Read the model definition and answer for the solid it produces. Units are mm, in the model's axes. A direction names the side the tool comes from. Give positions to 0.01 mm unless a question says otherwise; leave off trailing zeros. Order: outer loops, then holes, each group sorted by start corner. A loop starts at its lowest first (then second) coordinate and runs counter-clockwise, first axis right, second up. Notation, with made-up numbers: (77, 55) - (134, 55) arc R18 ccw to (134, 74) - close; hole circle Ø11 at (81.25, 71.25). An arc over 180 degrees is marked (long way). Use a Markdown table: item, result. Add a question column.
1. A cutting plane is placed at C-C on z = 39. Determine the outline of the cut face in (x, y), and give its area (3 significant figures).
2. Flat-ended cylindrical pins translate along their axes: P1, Ø2.5, axis at y = 5.5, z = 53.5, coming from the -X side; P2, Ø3, axis at x = 59, z = 24, coming from the +Y side; P3, Ø2, axis at x = 76.5, z = 18.5, coming from the +Y side. Find the tip coordinate at first contact, or state that the pin passes through.
3. A cutting plane is placed at D-D on y = 1.5. State how many separate pieces and enclosed holes the cut face has, and give its area (3 significant figures).
4. For a pull along X with two mould halves and no side action, classify faces 1 (the cylindrical face through (75.3, 5.3, 16.9)), 2 (the flat face through (2.487, 3, 2)), 3 (the flat face through (87.17, 3, 50)) as released by +X, released by -X, zero draft, split by the parting line, or undercut.
5. A cutting plane is placed at A-A on z = 25. Determine the outline of the cut face in (x, y).
6. A cutting plane is placed at B-B on x = 69. Determine the outline of the cut face in (y, z), and give its area (3 significant figures).
7. Consider L1, parallel to X at y = 1.5, z = 26; L2, parallel to Z at x = 14.5, y = 3; L3, parallel to X at y = 4.25, z = 18. Determine where each line is inside the solid, lowest interval first.
8. Which of the six approach directions +Z, -Z, +X, -X, +Y, -Y give full straight-line access (tool end or side, diameter ignored) to faces 4 (the flat face through (-27, 3, 46.102)), 5 (the flat face through (138.027, 3, 26)), 6 (the flat face through (87.17, 3, 2)), 7 (the flat face through (84.13, 3.13, 56.51)), 8 (the cylindrical face through (22.38, 3.92, 51.01))?
Autodesk Inventor part; units mm, degrees
ref_plane "YZ Plane" through (0, 0, 0) normal (1, 0, 0) x (0, 1, 0)
ref_plane "XZ Plane" through (0, 0, 0) normal (0, 1, 0) x (-1, 0, 0)
ref_plane "XY Plane" through (0, 0, 0) normal (0, 0, 1) x (1, 0, 0)
sketch "Sketch1" plane through (0, 0, 0) normal (0, 1, 0) x (-1, 0, 0)
  line L0 (-41.4486, 0) -> (-10.4831, 0)
  line L1 (-10.4831, 0) -> (-10.4831, 53.4636)
  line L2 (-10.4831, 53.4636) -> (-41.4486, 53.4636)
  line L3 (-41.4486, 53.4636) -> (-41.4486, 0)
  line L4 (-79.1688, 53.4636) -> (-87.1698, 53.4636)
  line L5 (-87.1698, 53.4636) -> (-87.1698, 0)
  line L6 (-87.1698, 0) -> (-79.1688, 0)
  line L7 (-79.1688, 0) -> (-79.1688, 53.4636)
  line L8 (-87.1698, 53.4636) -> (-2.487, 53.4636)
  line L9 (-2.487, 53.4636) -> (-2.487, 59.4685)
  line L10 (-2.487, 59.4685) -> (-87.1698, 59.4685)
  line L11 (-87.1698, 59.4685) -> (-87.1698, 53.4636)
  line L12 (-87.1698, 0) -> (-2.487, 0)
  line L13 (-2.487, 0) -> (-2.487, -7.9038)
  line L14 (-2.487, -7.9038) -> (-87.1698, -7.9038)
  line L15 (-87.1698, -7.9038) -> (-87.1698, 0)
  line L16 (-87.1698, -7.9038) -> (-2.487, -7.9038)
  line L17 (-2.487, -7.9038) -> (-2.487, 59.4685)
  line L18 (-2.487, 59.4685) -> (-87.1698, 59.4685)
  line L19 (-87.1698, 59.4685) -> (-87.1698, -7.9038)
  line L20 (-2.487, -7.9038) -> (-2.487, 25.802)
  line L21 (-2.487, 25.802) -> (-2.487, 59.4685)
  point P0 (0, 0)
  dimension "d0" = 8.001
  dimension "d1" = 33.7058
extrude "Extrusion1" add sketch "Sketch1" along normal blind 6.35
sketch "Sketch3" plane through (0, 6.35, 0) normal (0, 1, 0) x (1, 0, 0)
  line L0 (10.5148, -0.1125) -> (75.0308, -0.1125)
  line L1 (75.0308, -0.1125) -> (76.5548, -1.6365)
  line L2 (76.5548, -1.6365) -> (76.5548, -13.003)
  line L3 (76.5997, -13.1114) -> (79.0948, -15.6065)
  line L4 (79.0948, -15.6065) -> (79.0948, -48.3725)
  line L5 (79.0948, -48.3725) -> (76.5997, -50.8676)
  line L6 (76.5548, -50.976) -> (76.5548, -53.4525)
  line L7 (76.5548, -53.4525) -> (10.5148, -53.4525)
  line L8 (10.5148, -53.4525) -> (10.5148, -0.1125)
  line L9 (77.3168, -12.7509) -> (77.3168, -1.3209)
  line L10 (77.3168, -1.3209) -> (75.3465, 0.6495)
  line L11 (75.3465, 0.6495) -> (9.7528, 0.6495)
  line L12 (9.7528, 0.6495) -> (9.7528, -54.2145)
  line L13 (9.7528, -54.2145) -> (77.3168, -54.2145)
  line L14 (77.3168, -54.2145) -> (77.3168, -51.2282)
  line L15 (77.3168, -51.2282) -> (79.8568, -48.6882)
  line L16 (79.8568, -48.6882) -> (79.8568, -15.2909)
  line L17 (79.8568, -15.2909) -> (77.3168, -12.7509)
  point P0 (0, 0)
  dimension "d4" = 0.762
  dimension "d5" = 0.762
  dimension "d6" = 0.762
  dimension "d7" = 0.762
  dimension "d8" = 0.762
  dimension "d9" = 0.762
extrude "Extrusion2" cut sketch "Sketch3" against normal blind 3
sketch "Sketch4" plane through (0, 3.35, 0) normal (0, 1, 0) x (1, 0, 0)
  circle A0 centre (76.5548, -17.8925) radius 1.6 construction
  circle A1 centre (76.5548, -45.8325) radius 1.6 construction
  circle A2 centre (24.4848, -50.9125) radius 1.6 construction
  circle A3 centre (25.7548, -2.6525) radius 1.6 construction
  circle A4 centre (25.7548, -2.6525) radius 2.108
  circle A5 centre (76.5548, -17.8925) radius 2.108
  circle A6 centre (76.5548, -45.8325) radius 2.108
  circle A7 centre (24.4848, -50.9125) radius 2.108
  point P0 (0, 0)
  dimension "d12" = 0.508
  dimension "d13" = 0.508
  dimension "d14" = 0.508
  dimension "d15" = 0.508
extrude "Extrusion3" add sketch "Sketch4" along normal blind 1.1641
sketch "Sketch5" plane through (25.7548, 4.5141, 2.6525) normal (0, 1, 0) x (1, 0, 0)
  circle A0 centre (0, 0) radius 2.108
  circle A1 centre (0, 0) radius 1.6
  circle A2 centre (-1.27, -48.26) radius 2.108
  circle A3 centre (-1.27, -48.26) radius 2.108
  circle A4 centre (-1.27, -48.26) radius 1.6
  circle A5 centre (50.8, -43.18) radius 2.108
  circle A6 centre (50.8, -43.18) radius 2.108
  circle A7 centre (50.8, -15.24) radius 2.108
  circle A8 centre (50.8, -15.24) radius 2.108
  circle A9 centre (50.8, -15.24) radius 1.6
  circle A10 centre (50.8, -43.18) radius 1.6
  point P0 (-25.7548, 2.6525)
  dimension "d18" = 3.2
  dimension "d27" = 3.2
  dimension "d28" = 3.2
  dimension "d29" = 3.2
extrude "Extrusion4" add sketch "Sketch5" along normal blind 1.6002 contours A1 | A4 | A9 | A10
sketch "Sketch8" plane through (25.7548, 6.1143, 2.6525) normal (0, 1, 0) x (1, 0, 0)
  circle A0 centre (0, 0) radius 0.7658
  circle A1 centre (50.8, -15.24) radius 1.6
  circle A2 centre (50.8, -15.24) radius 0.7658
  circle A3 centre (50.8, -43.18) radius 1.6
  circle A4 centre (50.8, -43.18) radius 0.7658
  circle A5 centre (-1.27, -48.26) radius 1.6
  circle A6 centre (-1.27, -48.26) radius 0.7658
  point P0 (-25.7548, 2.6525)
  dimension "d32" = 1.5316
  dimension "d33" = 1.5316
  dimension "d34" = 1.5316
  dimension "d35" = 1.5316
extrude "Extrusion5" cut sketch "Sketch8" against normal blind 14.986 contours A0 | A2 | A4 | A6
sketch "Sketch9" plane through (0, 6.35, 0) normal (0, 1, 0) x (1, 0, 0)
  line L0 (87.1698, 7.9038) -> (2.487, 7.9038)
  line L1 (44.8284, 7.9038) -> (44.8284, -59.4685)
  line L2 (2.487, -59.4685) -> (87.1698, -59.4685)
  line L3 (2.487, 7.9038) -> (2.487, -59.4685)
  line L4 (2.487, -25.7823) -> (87.1698, -25.7823)
  line L5 (87.1698, -59.4685) -> (87.1698, 7.9038)
  line L6 (2.487, -25.7823) -> (-55.933, -25.7823)
  line L7 (-55.933, -25.7823) -> (-55.933, -5.4623)
  line L8 (-55.933, -5.4623) -> (2.487, -5.4623)
  line L9 (2.487, -5.4623) -> (2.487, -25.7823)
  line L10 (-55.933, -25.7823) -> (-55.933, -46.1023)
  line L11 (-55.933, -46.1023) -> (2.487, -46.1023)
  circle A0 centre (14.7725, 4.3917) radius 1.524
  line L12 (145.5898, -25.7823) -> (145.5898, -5.4623)
  line L13 (145.5898, -5.4623) -> (87.1698, -5.4623)
  line L14 (145.5898, -25.7823) -> (145.5898, -46.1023)
  line L15 (145.5898, -46.1023) -> (87.1698, -46.1023)
  circle A1 centre (74.8844, 4.3917) radius 1.524
  circle A2 centre (14.7725, -55.9564) radius 1.524
  circle A3 centre (74.8844, -55.9564) radius 1.524
  line L16 (87.1698, -46.1023) -> (87.1698, -5.4623)
  line L17 (2.487, -46.1023) -> (2.487, -5.4623)
  circle A4 centre (14.7725, -55.9564) radius 1.524
  circle A5 centre (14.7725, 4.3917) radius 1.524
  circle A6 centre (74.8844, 4.3917) radius 1.524
  point P0 (0, 0)
  dimension "d38" = 58.42
  dimension "d39" = 20.32
  dimension "d40" = 3.048
extrude "Extrusion6" add sketch "Sketch9" against normal blind 6.35 contours L13 L12 L14 L15 L5 | L3 L6 L7 L8 | L3 L11 L10 L6
sketch "Sketch10" plane through (0, 6.35, 0) normal (0, 1, 0) x (1, 0, 0)
  point P0 (0, 0)
extrude "Extrusion7" cut sketch "Sketch9" against normal blind 9.906 contours A0 | A1 | A2 | A3
sketch "Sketch11" plane through (0, 6.35, 0) normal (0, 1, 0) x (1, 0, 0)
  line L0 (-55.933, -46.1023) -> (-55.933, -5.4623)
  line L1 (-55.933, -25.7823) -> (145.5898, -25.7823)
  line L2 (145.5898, -5.4623) -> (145.5898, -46.1023)
  line L3 (87.1698, 7.9038) -> (2.487, 7.9038)
  line L4 (44.8284, 7.9038) -> (44.8284, -59.4685)
  line L5 (2.487, -59.4685) -> (87.1698, -59.4685)
  line L6 (-55.933, -25.7823) -> (-26.469, -25.7823)
  line L7 (-26.469, -25.7823) -> (-26.469, -19.5593)
  line L8 (-26.469, -19.5593) -> (-55.933, -19.5593)
  line L9 (-55.933, -19.5593) -> (-55.933, -25.7823)
  line L10 (-26.469, -25.7823) -> (-55.933, -25.7823)
  line L11 (-55.933, -25.7823) -> (-55.933, -32.0067)
  line L12 (-55.933, -32.0067) -> (-26.469, -32.0067)
  line L13 (-26.469, -32.0067) -> (-26.469, -25.7823)
  line L14 (-55.933, -25.7823) -> (-26.469, -25.7823)
  line L15 (-26.469, -25.7823) -> (-26.469, -32.0067)
  line L16 (-26.469, -32.0067) -> (-55.933, -32.0067)
  line L17 (-55.933, -32.0067) -> (-55.933, -25.7823)
  line L18 (-55.933, -19.5593) -> (-38.633, -19.5593)
  line L19 (-55.933, -25.7823) -> (-55.933, -18.2823)
  line L20 (-55.933, -18.2823) -> (-38.633, -18.2823)
  line L21 (-38.633, -18.2823) -> (-38.633, -12.4823)
  line L22 (-38.633, -12.4823) -> (-47.133, -12.4823)
  line L23 (-47.133, -12.4823) -> (-47.133, -18.2823)
  line L24 (-48.3704, -25.7823) -> (-48.3704, -18.1623)
  line L25 (-48.3704, -18.1623) -> (-50.9104, -18.1623)
  line L26 (-50.9104, -18.1623) -> (-50.9104, -25.7823)
  line L27 (-42.883, -25.7823) -> (-42.883, -16.7823)
  circle A0 centre (-42.883, -16.7823) radius 0.8001
  line L28 (-48.3704, -25.7823) -> (-48.3704, -33.4023)
  line L29 (-48.3704, -33.4023) -> (-50.9104, -33.4023)
  line L30 (-50.9104, -33.4023) -> (-50.9104, -25.7823)
  circle A1 centre (-42.883, -34.7823) radius 0.8001
  line L31 (138.0273, -25.7823) -> (138.0273, -18.1623)
  line L32 (138.0273, -18.1623) -> (140.5673, -18.1623)
  line L33 (140.5673, -18.1623) -> (140.5673, -25.7823)
  circle A2 centre (132.5398, -16.7823) radius 0.8001
  circle A3 centre (132.5398, -34.7823) radius 0.8001
  line L34 (138.0273, -25.7823) -> (138.0273, -33.4023)
  line L35 (140.5673, -33.4023) -> (140.5673, -25.7823)
  line L36 (138.0273, -33.4023) -> (140.5673, -33.4023)
  point P0 (0, 0)
  dimension "d64" = 2
  dimension "d45" = 29.464
  dimension "d46" = 6.223
  dimension "d47" = 17.3
  dimension "d48" = 7.5
  dimension "d49" = 5.8
  dimension "d50" = 8.5
  dimension "d51" = 7.62
  dimension "d52" = 2.54
  dimension "d53" = 9
  dimension "d54" = 1.6002
extrude "Extrusion8" cut sketch "Sketch11" against normal blind 25.4 contours L31 L32 L33 L1 | L1 L35 L36 L34 | L30 L1 L28 L12 | L12 L28 L29 L30 | L26 L8 L24 L1 | L26 L20 L24 L8 | L26 L25 L24 L20 | A0 | A1 | A2 | A3
sketch "Sketch12" plane through (87.1698, 0, -7.9038) normal (0, 0, -1) x (-1, 0, 0)
  point P0 (87.1698, 0)
sketch "Sketch13" plane through (-55.933, 6.35, 8.6373) normal (-1, 0, 0) x (0, 0, 1)
  point P0 (-8.6373, -6.35)
sketch "Sketch15" plane through (0, 3.35, 0) normal (0, 1, 0) x (1, 0, 0)
  line L0 (-55.933, -5.4623) -> (-55.933, -46.1023)
  line L1 (-55.933, -25.7823) -> (145.5898, -25.7823)
  line L2 (145.5898, -5.4623) -> (145.5898, -46.1023)
  point P0 (0, 0)
  point P1 (-55.933, -8.6373)
  point P2 (-55.933, -42.9273)
  point P3 (145.5898, -8.6373)
  point P4 (145.5898, -42.9273)
  dimension "d61" = 201.5228
sketch "Sketch16" plane through (-55.933, 6.35, 8.6373) normal (-1, 0, 0) x (0, 0, 1)
  line L0 (45.5772, 0) -> (-9.2868, 0)
  line L1 (18.1452, 0) -> (18.1452, -6.35)
  line L2 (9.525, -6.35) -> (24.765, -6.35)
  point P0 (-8.6373, -6.35)
  dimension "d62" = 6.35
chamfer "Chamfer2" distance 6 angle 45 4 edges at (87.1698, 3.175, -7.9038) (87.1698, 3.175, 59.4685) (2.487, 3.175, 59.4685) (2.487, 3.175, -7.9038)
equation "\"d4\" = d5"
equation "\"d6\" = d5"
equation "\"d7\" = d5"
equation "\"d8\" = d5"
equation "\"d9\" = d5"
equation "\"d13\" = d12"
equation "\"d14\" = d12"
equation "\"d15\" = d12"
properties part number "base"
Output values:
| question | item | result |
|---|---|---|
| 1 | outline | (-55.93, 0) - (145.59, 0) - (145.59, 6.35) - (79.86, 6.35) - (79.86, 3.35) - (9.75, 3.35) - (9.75, 6.35) - (-55.93, 6.35) - close |
| 1 | area | 1,070 mm² |
| 2 | P1 | x = 2.49 |
| 2 | P2 | y = 3.35 |
| 2 | P3 | y = 6.11 |
| 3 | separate pieces | 1 |
| 3 | enclosed holes | 14 |
| 3 | area | 10,300 mm² |
| 4 | face 1 | undercut |
| 4 | face 2 | released by -X |
| 4 | face 3 | released by +X |
| 5 | outline | (-55.93, 0) - (-50.91, 0) - (-50.91, 6.35) - (-55.93, 6.35) - close; (-48.37, 0) - (138.03, 0) - (138.03, 6.35) - (79.86, 6.35) - (79.86, 3.35) - (9.75, 3.35) - (9.75, 6.35) - (-48.37, 6.35) - close; (140.57, 0) - (145.59, 0) - (145.59, 6.35) - (140.57, 6.35) - close |
| 6 | outline | (0, -7.9) - (6.35, -7.9) - (6.35, -0.65) - (3.35, -0.65) - (3.35, 54.21) - (6.35, 54.21) - (6.35, 59.47) - (0, 59.47) - close |
| 6 | area | 263 mm² |
| 7 | L1 | -55.93 to -50.91, -48.37 to 138.03, 140.57 to 145.59 |
| 7 | L2 | -7.9 to -5.89, -2.89 to 54.46, 57.46 to 59.47 |
| 7 | L3 | -55.93 to 9.75, 74.45 to 75.8, 77.31 to 78.66, 79.86 to 145.59 |
| 8 | face 4 | +Z, -X, +Y, -Y |
| 8 | face 5 | +Y, -Y |
| 8 | face 6 | -Z, +X, +Y, -Y |
| 8 | face 7 | +Z, +X, +Y, -Y |
| 8 | face 8 | +Y |
